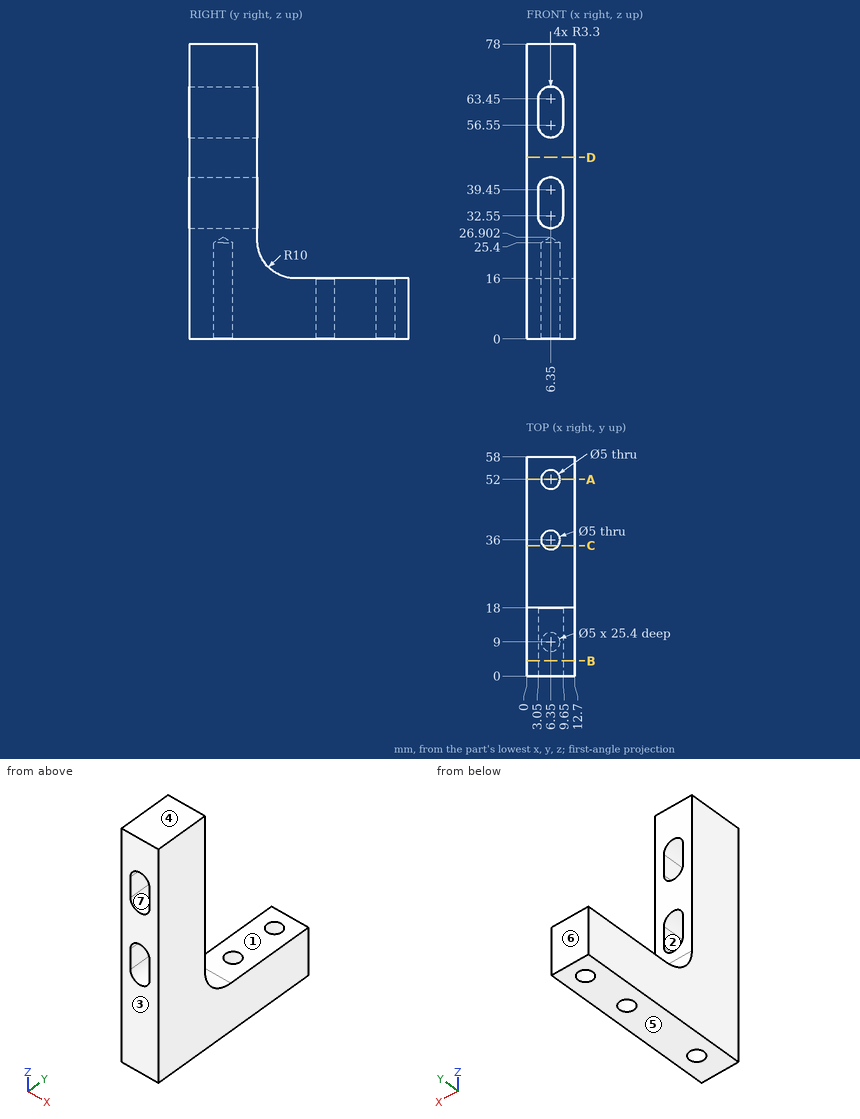
For this review, use the dimensioned drawing (mm, ordinates from the lowest corner) and the shaded views. A direction names the side the tool comes from. Round coordinates to 2 decimals unless told otherwise and drop trailing zeros. Order: outer loops, then holes, each group sorted by start corner. A loop starts at its lowest first (then second) coordinate and runs counter-clockwise, first axis right, second up. Notation, with made-up numbers: M 87.5,0.5 L 98.5,0.5 A28 cw 98.5,22.5 Z; hole C -14.75,25.5 d3. An arc over 180 degrees is marked long. Write each question's results on one line, items separated by ' | '. Start each with the question number.
1. Draft analysis for pull direction Z (two halves, no side actions). For the marked faces 4, 5, 6 and 7, state which applies: pulls with the +Z half, pulls with the -Z half, needs draft (parallel to the pull), parting line crosses it, or undercut.
2. To check wall thickness, follow L1, parallel to Y at x = 6.35, z = 7.25; L2, parallel to X at y = 9, z = 8.5; L3, parallel to Z at x = 7.25, y = 5 (1 decimal). State the ranges of each line that lie inside material, in increasing order. Write a range as [from, to].
3. Add section B-B (y = 4). State the section outline as (x, z) points, then the cut area to 3 significant figures.
4. Tool access review of the marked faces 1, 2 and 3: name each direction out of +Z, -Z, +X, -X, +Y, -Y from which nothing blocks a thin tool from reaching the whole face with its end or side.
5. Clearance check with flat-ended pins moving along their axes: pin 1 Ø7.5 at (y, z) = (7, 36) entering from -X; pin 2 Ø6 at (x, z) = (3.5, 36.5) entering from +Y. State where each tip first meets the part, or that it passes through.
6. Add section A-A (y = 52). State the section outline as (x, z) points, then the cut area to 3 significant figures.
7. Add section C-C (y = 34.5). State the section outline as (x, z) points.
8. Add section D-D (z = 48). State the section outline as (x, y) points, then the cut area to 3 significant figures.
Output values:
1) face 4: pulls with the +Z half | face 5: pulls with the -Z half | face 6: needs draft | face 7: undercut
2) L1: [0, 6.5], [11.5, 33.5], [38.5, 49.5], [54.5, 58] | L2: [0, 3.85], [8.85, 12.7] | L3: [0, 29.4], [42.6, 53.4], [66.6, 78]
3) outline: M 0,0 L 12.7,0 L 12.7,78 L 0,78 Z; hole M 3.05,32.55 A3.3 ccw 9.65,32.55 L 9.65,39.45 A3.3 ccw 3.05,39.45 Z; hole M 3.05,56.55 A3.3 ccw 9.65,56.55 L 9.65,63.45 A3.3 ccw 3.05,63.45 Z | area: 831 mm^2
4) face 1: +Z, +X, -X, +Y | face 2: +Y, -Y | face 3: +Z, -Z, +X, -X, -Y
5) pin 1: x = 0 | pin 2: y = 18
6) outline: M 0,0 L 3.85,0 L 3.85,16 L 0,16 Z; M 8.85,0 L 12.7,0 L 12.7,16 L 8.85,16 Z | area: 123 mm^2
7) outline: M 0,0 L 4.35,0 L 4.35,16 L 0,16 Z; M 8.35,0 L 12.7,0 L 12.7,16 L 8.35,16 Z
8) outline: M 0,0 L 12.7,0 L 12.7,18 L 0,18 Z | area: 229 mm^2
